```python
from build123d import *

# Parameters (mm, degrees)
SKETCH1_W           = 6.50875
SKETCH1_H           = 5.715
SKETCH1_W_2         = 3.96875
SKETCH1_H_2         = 3.175
BOSS_EXTRUDE1_DEPTH = 25.4
SKETCH2_W           = 41.275
SKETCH2_H           = 41.275
SKETCH2_W_2         = 6.50875
SKETCH2_H_2         = 5.715
BOSS_EXTRUDE2_DEPTH = 2.54
CUT_EXTRUDE1_DEPTH  = 39.690732902
FILLET1_R           = 2.54


with BuildPart() as part:
    # Sketch1 → Boss-Extrude1 (new body)
    with BuildSketch(Plane(origin=(0, 0, 0), x_dir=(1, 0, 0), z_dir=(0, 1, 0))):
        Rectangle(SKETCH1_W, SKETCH1_H)
        Rectangle(SKETCH1_W_2, SKETCH1_H_2, mode=Mode.SUBTRACT)
    extrude(amount=BOSS_EXTRUDE1_DEPTH)

    # Sketch2 → Boss-Extrude2 (add)
    with BuildSketch(Plane(origin=(0, 25.4, 0), x_dir=(1, 0, 0), z_dir=(0, 1, 0))):
        Rectangle(SKETCH2_W, SKETCH2_H)
        Rectangle(SKETCH2_W_2, SKETCH2_H_2, mode=Mode.SUBTRACT)
    extrude(amount=-BOSS_EXTRUDE2_DEPTH)

    # Sketch3 → Cut-Extrude1 (cut, through all)
    with BuildSketch(Plane(origin=(0, 25.4, 0), x_dir=(1, 0, 0), z_dir=(0, 1, 0))):
        Polygon((-2.122897552, 5.715), (-14.505397552, 18.0975), (14.505397552, 18.0975), (2.122897552, 5.715), align=None)
        Polygon((-5.715, 2.122897552), (-18.0975, 14.505397552), (-18.0975, -14.505397552), (-5.715, -2.122897552), align=None)
        Polygon((-14.505397552, -18.0975), (-2.122897552, -5.715), (2.122897552, -5.715), (14.505397552, -18.0975), align=None)
        Polygon((18.0975, 14.505397552), (5.715, 2.122897552), (5.715, -2.122897552), (18.0975, -14.505397552), align=None)
    extrude(amount=-CUT_EXTRUDE1_DEPTH, mode=Mode.SUBTRACT)

    # Fillet1
    fillet1_edges = [part.edges().sort_by_distance(p)[0] for p in [
        (20.6375, 24.13, -20.6375),
        (20.6375, 24.13, 20.6375),
        (-20.6375, 24.13, 20.6375),
        (-20.6375, 24.13, -20.6375),
    ]]
    fillet(fillet1_edges, radius=FILLET1_R)


solid = part.part
```
Model file for the job. Use its own axes, mm. A direction names the side the tool comes from. Coordinates: 2 decimals unless noted, no trailing zeros. Loops run counter-clockwise (first coordinate to the right, second up) from the corner with the lowest first, then second, coordinate; pieces in that order, holes last. Notation, with made-up numbers: (23.25, -12.5) - (27.25, -12.5) arc R25 ccw to (27.25, 16.5) - close; hole circle Ø2 at (-2.75, 34). An arc over 180 degrees is marked (long way). Answer as a JSON object with one key per item and string values. Group by question number.
(1) Cut at A-A (x = -1). Give the cut face in (y, z) (1 decimal).
(2) Two-plate mould, pull along X, no slides. Class faces 6 (the face through (-3.254, 11, 0)), 7 (the face through (1.984, 13, 0)), 8 (the face through (-11.99, 24.15, 8.4)), 9 (the face through (0, 24, -20.638)): released by +X, released by -X, zero draft, split by the parting line, or undercut.
(3) Cut at D-D (y = 19). Give the cut face in (x, z), then the cut area to 3 significant figures.
(4) Flat gauge pins, fed straight in: pin 1 (1.2 mm diameter, centred on x = -1, y = 18, fed in from -Z); pin 2 (12 mm diameter, centred on y = 5.5, z = 6.5, fed in from +X); pin 3 (7 mm diameter, centred on x = 0, y = 11, fed in from +Z); pin 4 (4 mm diameter, centred on y = 21.5, z = 6, fed in from -X). Where does each tip first touch, or does it go through?
(5) Cut at B-B (z = -5). Give the cut face in (x, y).
(6) Probe line 1 along X through (y, z) = (11.75, 0); line 2 along Z through (x, y) = (10, 24); line 3 along Y through (x, z) = (-10, 13). List the from-to ranges inside material, lowest first.
(7) Cut at C-C (z = -16.5). Give the cut face in (x, y).
(8) Tool access for faces 1 (the face through (3.254, 11, 0)), 2 (the face through (-19.913, 24.112, 19.874)), 3 (the face through (0, 11, -2.858)), 4 (the face through (18.098, 24, 0)), 5 (the face through (0, 0, -2)): list every direction of +Z, -Z, +X, -X, +Y, -Y with a clear straight run to the whole face (end or side of a thin tool).
Geometry says:
{
 "1": {"outline": "(0, -2.9) - (22.9, -2.9) - (22.9, -5.7) - (25.4, -5.7) - (25.4, -1.6) - (0, -1.6) - close; (0, 1.6) - (25.4, 1.6) - (25.4, 5.7) - (22.9, 5.7) - (22.9, 2.9) - (0, 2.9) - close; (22.9, -20.6) - (25.4, -20.6) - (25.4, -18.1) - (22.9, -18.1) - close; (22.9, 18.1) - (25.4, 18.1) - (25.4, 20.6) - (22.9, 20.6) - close"},
 "2": {"face 6": "released by -X", "face 7": "undercut", "face 8": "undercut", "face 9": "zero draft"},
 "3": {"outline": "(-3.25, -2.86) - (3.25, -2.86) - (3.25, 2.86) - (-3.25, 2.86) - close; hole (-1.98, -1.59) - (1.98, -1.59) - (1.98, 1.59) - (-1.98, 1.59) - close", "area": "24.6 mm^2"},
 "4": {"pin 1": "stops at z = -2.86", "pin 2": "stops at x = 3.25", "pin 3": "stops at z = 2.86", "pin 4": "stops at x = -20.64"},
 "5": {"outline": "(-20.64, 22.86) - (-18.1, 22.86) - (-18.1, 25.4) - (-20.64, 25.4) - close; (-8.59, 22.86) - (8.59, 22.86) - (8.59, 25.4) - (-8.59, 25.4) - close; (18.1, 22.86) - (20.64, 22.86) - (20.64, 25.4) - (18.1, 25.4) - close"},
 "6": {"line 1": "x = -3.25 to -1.98, 1.98 to 3.25", "line 2": "z = -20.64 to -18.1, -13.59 to -6.41, 6.41 to 13.59, 18.1 to 20.64", "line 3": "y = 22.86 to 25.4"},
 "7": {"outline": "(-20.64, 22.86) - (-12.91, 22.86) - (-12.91, 25.4) - (-20.64, 25.4) - close; (12.91, 22.86) - (20.64, 22.86) - (20.64, 25.4) - (12.91, 25.4) - close"},
 "8": {"face 1": "+Z, -Z, +X, -Y", "face 2": "+Z, -X, +Y, -Y", "face 3": "-Z, +X, -X, -Y", "face 4": "+Y, -Y", "face 5": "+Z, -Z, +X, -X, -Y"}
}
